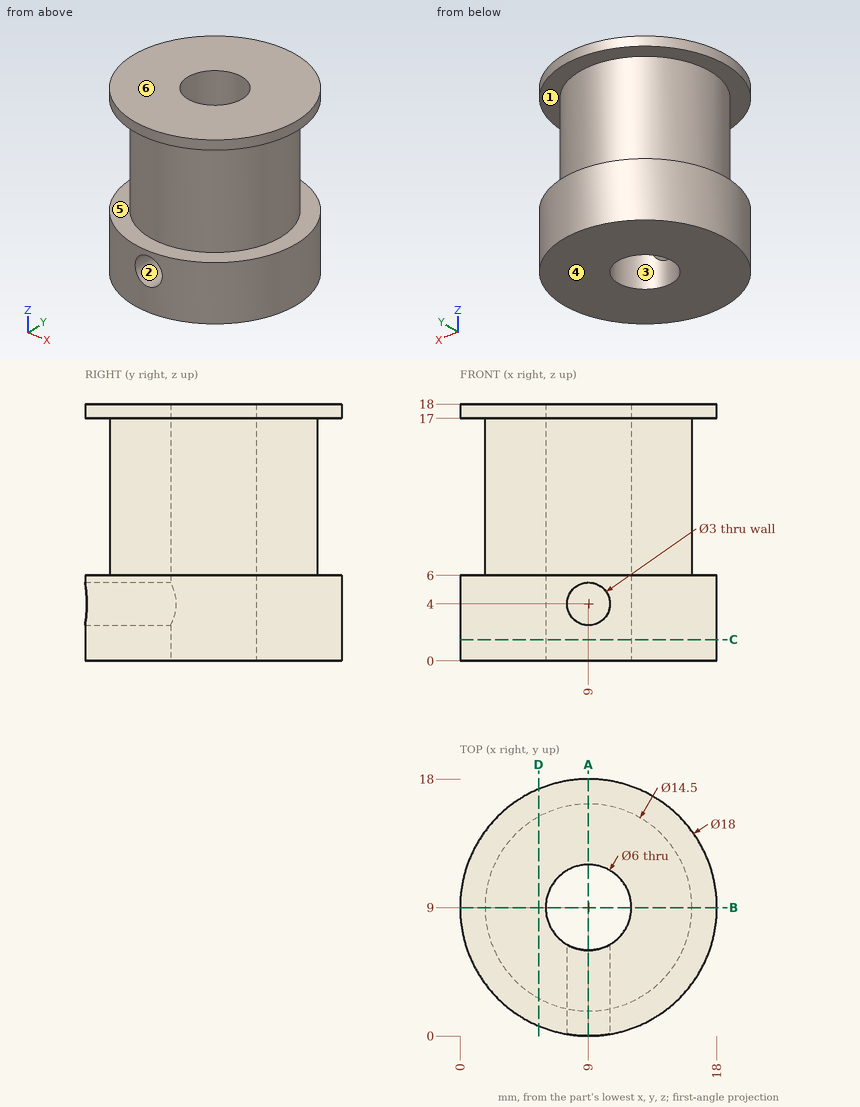
For this review, use the dimensioned drawing (mm, ordinates from the lowest corner) and the shaded views. A direction names the side the tool comes from. Give positions to 0.01 mm unless a question says otherwise; leave off trailing zeros. Order: outer loops, then holes, each group sorted by start corner. A loop starts at its lowest first (then second) coordinate and runs counter-clockwise, first axis right, second up.
1) Wall thickness on line 1 (Z direction, x = 9, y = 4.5); line 2 (Z direction, x = 15.75, y = 6); line 3 (Y direction, x = 9, z = 9): over which ranges is each line inside the solid? List them lowest first.
2) For the marked faces 1, 2 and 3, list the 3-axis set-ups (+Z, -Z, +X, -X, +Y, -Y) from which the entire face can be reached by the end or side of a thin tool; tool diameter is ignored.
3) Take a section at C-C (z = 1.5). Give the boundary of the cut face in (x, y).
4) The part is to be moulded in two halves that separate along Z. For the marked faces 4, 5 and 6, say which applies: released by +Z, released by -Z, zero draft, split by the parting line, or undercut.
5) Take a section at B-B (y = 9). Give the boundary of the cut face in (x, z).
6) Take a section at D-D (x = 5.5). Give the boundary of the cut face in (y, z), then the cut area to 3 significant figures.
7) Insertion check: pin 1 (8 mm diameter, centred on y = 16, z = 7, fed in from -X); pin 2 (3.5 mm diameter, centred on x = 9, y = 9, fed in from +Z); pin 3 (4 mm diameter, centred on y = 14, z = 6, fed in from -X); pin 4 (3 mm diameter, centred on y = 11.5, z = 4, fed in from +X). Each pin has a flat end and moves straight along its axis. Give the tip position at first contact, or say it passes through.
8) Take a section at A-A (x = 9). Give the boundary of the cut face in (y, z).
Derived:
1. line 1: z = 0 to 2.5, 5.5 to 18
1. line 2: z = 0 to 6, 17 to 18
1. line 3: y = 1.75 to 6, 12 to 16.25
2. face 1: none
2. face 2: -Y
2. face 3: +Z, -Z
3. outline: circle Ø18 at (9, 9); hole circle Ø6 at (9, 9)
4. face 4: released by -Z
4. face 5: undercut
4. face 6: released by +Z
5. outline: (0, 0) - (6, 0) - (6, 18) - (0, 18) - (0, 17) - (1.75, 17) - (1.75, 6) - (0, 6) - close; (12, 0) - (18, 0) - (18, 6) - (16.25, 6) - (16.25, 17) - (18, 17) - (18, 18) - (12, 18) - close
6. outline: (0.71, 0) - (17.29, 0) - (17.29, 6) - (15.35, 6) - (15.35, 17) - (17.29, 17) - (17.29, 18) - (0.71, 18) - (0.71, 17) - (2.65, 17) - (2.65, 6) - (0.71, 6) - close
6. area: 256 mm2
7. pin 1: stops at x = 0.56
7. pin 2: passes through
7. pin 3: stops at x = 0.51
7. pin 4: stops at x = 17.94
8. outline: (0, 0) - (6, 0) - (6, 2.5) - (0, 2.5) - close; (0, 5.5) - (6, 5.5) - (6, 18) - (0, 18) - (0, 17) - (1.75, 17) - (1.75, 6) - (0, 6) - close; (12, 0) - (18, 0) - (18, 6) - (16.25, 6) - (16.25, 17) - (18, 17) - (18, 18) - (12, 18) - close
